Model file for the job. Use its own axes, mm. Face numbers are marked on the shaded views. Coordinates: 2 decimals unless noted, no trailing zeros. Loops run counter-clockwise (first coordinate to the right, second up) from the corner with the lowest first, then second, coordinate; pieces in that order, holes last.
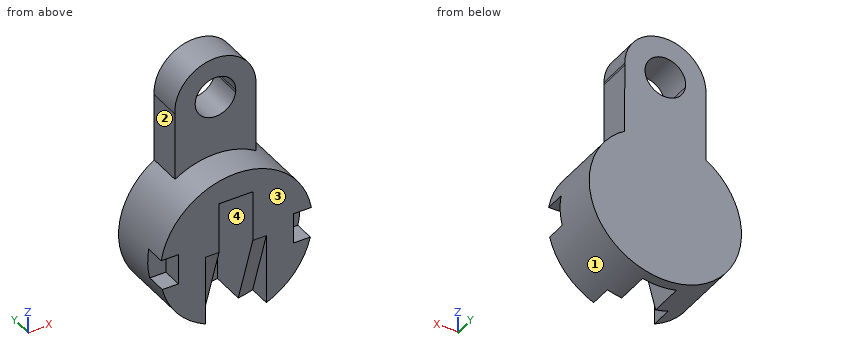
from build123d import *

# Parameters (mm, degrees)
F0_R      = 22.5
F1_DEPTH  = 20
F2_W      = 2.5675058744
F2_H      = 9
F3_DEPTH  = 6
F5_DEPTH  = 17
F7_DEPTH  = 4
F9_DEPTH  = 4
F11_DEPTH = 10


with BuildPart() as f1:
    # F0 (on Front) → F1 (new body)
    with BuildSketch(Plane.XZ):
        Circle(F0_R)
    extrude(amount=F1_DEPTH)

    # F2 (on face) → F3 (cut)
    with BuildSketch(Plane.XZ.offset(20)):
        with BuildLine():
            Line((-19.6791486824, 3.7585074455), (-22.183859488, 3.7585074455))
            ThreePointArc((-22.183859488, 3.7585074455), (-22.4872686861, -0.7568005275), (-21.8809678899, -5.2414925545))
            Line((-21.8809678899, -5.2414925545), (-19.6791486824, -5.2414925545))
            Line((-19.6791486824, -5.2414925545), (-19.6791486824, 3.7585074455))
        make_face()
        with Locations((-18.3953957452, -0.7414925545)):
            Rectangle(F2_W, F2_H)
        with BuildLine():
            ThreePointArc((22.5, 0), (22.42082557, 1.885889912), (22.183859488, 3.7585074455))
            Line((22.183859488, 3.7585074455), (16.888357192, 3.7585074455))
            Line((16.888357192, 3.7585074455), (16.888357192, -5.2414925545))
            Line((16.888357192, -5.2414925545), (21.8809678899, -5.2414925545))
            ThreePointArc((21.8809678899, -5.2414925545), (22.3447060567, -2.638960257), (22.5, 0))
        make_face()
    extrude(amount=-F3_DEPTH, mode=Mode.SUBTRACT)

    # F4 (on face) → F5 (cut)
    with BuildSketch(Plane.XZ.offset(20)):
        with BuildLine():
            ThreePointArc((-5.111642808, -21.9116660207), (-0.1145059859, -22.4997086288), (4.888357192, -21.962558229))
            Line((4.888357192, -21.962558229), (4.888357192, 15))
            Line((4.888357192, 15), (-5.111642808, 15))
            Line((-5.111642808, 15), (-5.111642808, -21.9116660207))
        make_face()
    extrude(amount=-F5_DEPTH, mode=Mode.SUBTRACT)

    # F6 (on face) → F7 (cut)
    with BuildSketch(Plane(origin=(4.888357192, 0, 0), x_dir=(0, -1, 0), z_dir=(-1, 0, 0))):
        Polygon((20, 0), (13, -21.962558229), (20, -21.962558229), align=None)
    extrude(amount=-F7_DEPTH, mode=Mode.SUBTRACT)

    # F8 (on face) → F9 (cut)
    with BuildSketch(Plane.YZ.offset(-5.111642808)):
        Polygon((-20, -21.9116660207), (-13, -21.9116660207), (-20, 0), align=None)
    extrude(amount=-F9_DEPTH, mode=Mode.SUBTRACT)

    # F10 (on Front) → F11 (join)
    with BuildSketch(Plane.XZ):
        with BuildLine():
            ThreePointArc((11.9820211506, 39.3433652862), (0.0967969112, 28.0003904081), (-11.9698688592, 39.1501532526))
            Line((-11.9698688592, 39.1501532526), (-11.9698688592, 18.8409157593))
            Line((-11.9698688592, 18.8409157593), (12.0301311408, 18.8409157593))
            Line((12.0301311408, 18.8409157593), (11.9820211506, 39.3433652862))
        make_face()
        with BuildLine():
            ThreePointArc((5.958410645, 39.2947747978), (0.0483984556, 34.0001952041), (-5.9462583536, 39.1987437411))
            Line((-5.9462583536, 39.1987437411), (-11.9698688592, 39.1501532526))
            ThreePointArc((-11.9698688592, 39.1501532526), (0.0967969112, 28.0003904081), (11.9820211506, 39.3433652862))
            Line((11.9820211506, 39.3433652862), (5.958410645, 39.2947747978))
        make_face()
        with BuildLine():
            ThreePointArc((-5.9462583536, 39.1987437411), (-0.4015282546, 45.9865495121), (6, 40))
            ThreePointArc((6, 40), (5.9895936369, 39.6467747672), (5.958410645, 39.2947747978))
            Line((5.958410645, 39.2947747978), (11.9820211506, 39.3433652862))
            ThreePointArc((11.9820211506, 39.3433652862), (11.9955044456, 39.6715595996), (12, 40))
            ThreePointArc((12, 40), (-0.4251903631, 51.992464849), (-11.9698688592, 39.1501532526))
            Line((-11.9698688592, 39.1501532526), (-5.9462583536, 39.1987437411))
        make_face()
    extrude(amount=F11_DEPTH)


solid = f1.part
Q1. Slice it at D-D (x = -11). List the corners of the cut face in (y, z), and give its area (3 significant figures).
Answers:
outline: (-20, -19.63) - (0, -19.63) - (0, 44.8) - (-10, 44.8) - (-10, 19.63) - (-20, 19.63) - close
area: 1,040 mm2
Q2. Mould opens along X. For the marked faces 1, 2, 3 and 4 say: +X half, -X half, draft (parallel to the pull), parting line (faces both ways), or undercut.
Answers:
face 1: parting line
face 2: -X half
face 3: draft
face 4: undercut
Q3. Slice it at B-B (x = 7). List the corners of the cut face in (y, z).
Answers:
outline: (-20, 0) - (-13.18, -21.38) - (0, -21.38) - (0, 49.75) - (-10, 49.75) - (-10, 21.38) - (-20, 21.38) - close
Q4. Flat gauge pins, fed straight in: P1, Ø10, axis at y = -2.5, z = 29, coming from the +X side; P2, Ø1.6, axis at x = -20.5, z = -2, coming from the -Y side; P3, Ø5.5, axis at y = -16.5, z = -9.5, coming from the +X side; P4, Ø7, axis at x = 0, z = 38.5, coming from the -Y side. Where does each tip first touch, or does it go through?
Answers:
P1: stops at x = 12.02
P2: stops at y = -14
P3: stops at x = 21.46
P4: passes through
Q5. Slice it at A-A (x = 0). List the corners of the cut face in (y, z).
Answers:
outline: (-20, 15) - (-3, 15) - (-3, -22.5) - (0, -22.5) - (0, 34) - (-10, 34) - (-10, 22.5) - (-20, 22.5) - close; (-10, 46) - (0, 46) - (0, 52) - (-10, 52) - close
Q6. Slice it at C-C (y = -11.5). List the corners of the cut face in (x, z).
Answers:
outline: (-5.11, -21.91) - (-5.11, 15) - (4.89, 15) - (4.89, -21.96) arc R22.5 ccw (long way) to start
Q7. Drill centre lines: line 1 (Z direction, x = 0, y = -6.25); line 2 (X direction, y = -4.5, z = 43.5); line 3 (X direction, y = -14, z = 7.5). Where is each one in solid material? Low to high.
Answers:
line 1: z = 15 to 34, 46 to 52
line 2: x = -11.48 to -4.87, 4.87 to 11.48
line 3: x = -21.21 to -5.11, 4.89 to 21.21
